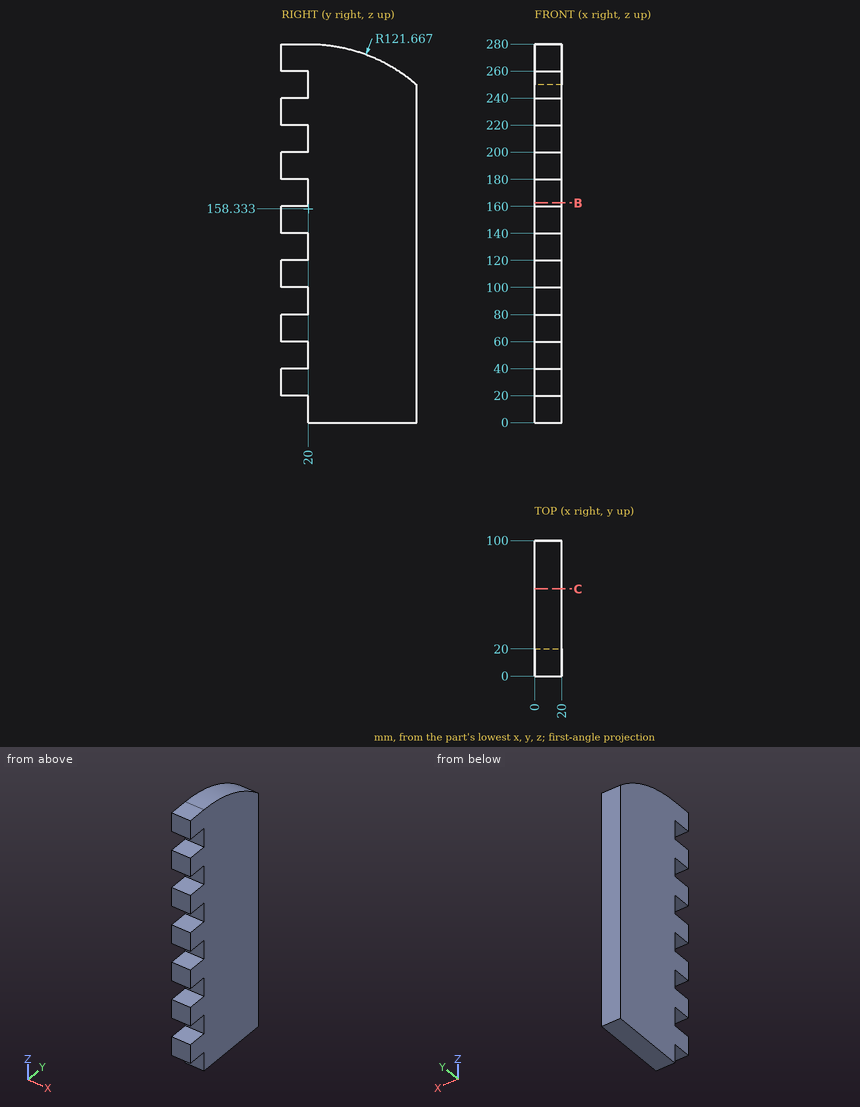
Input: dimensioned drawing with shaded views. Units: mm. Origin: part minimum x, y, z. Give positions to 0.01 mm unless a question says otherwise; leave off trailing zeros. Order: outer loops, then holes, each group sorted by start corner. A loop starts at its lowest first (then second) coordinate and runs counter-clockwise, first axis right, second up.
(1) Contact query for flat-ended pins moving along their axis: P1, Ø10, axis at x = 14.5, y = 14, coming from the -Z side; P2, Ø3, axis at x = 6.5, z = 203, coming from the -Y side; P3, Ø6, axis at x = 6.5, y = 39.5, coming from the +Z side. Output: stop coordinate, or through.
(2) Section query C-C (y = 64.5). Return the cut outline in (x, z), plus the area to 3 significant figures.
(3) Material intervals for line 1 along Y through (x, z) = (14.5, 50); line 2 along Z through (x, y) = (4.75, 21.5); line 3 along Z through (x, y) = (7.5, 57.5), sorted ascending.
(4) Section query B-B (z = 162.5). Return the cut outline in (x, y).
Outcome:
1. P1: stops at z = 20
1. P2: stops at y = 20
1. P3: stops at z = 278.88
2. outline: (0, 0) - (20, 0) - (20, 271.57) - (0, 271.57) - close
2. area: 5,430 mm2
3. line 1: y = 20 to 100
3. line 2: z = 0 to 279.99
3. line 3: z = 0 to 274.08
4. outline: (0, 20) - (20, 20) - (20, 100) - (0, 100) - close
